Geometry: final body of the model. Coordinates: model frame, mm. A direction names the side the tool comes from. Coordinates: 2 decimals unless noted, no trailing zeros. Loops run counter-clockwise (first coordinate to the right, second up) from the corner with the lowest first, then second, coordinate; pieces in that order, holes last. Notation, with made-up numbers: (3.25, -5.75) -> (11.25, -5.75) arc R18 ccw to (11.25, 9.25) -> close; hole circle Ø10 at (-40, 4.25). An arc over 180 degrees is marked (long way). One line per item, written item: value. Start each with the question number.
Item 1: Ray query, probe 1 along Y at (x, z) = (252, -203); probe 2 along Z at (x, y) = (253.1, 44.45); probe 3 along Z at (x, y) = (-142, 14). Return the intervals inside material, ascending. Write a range as from..to.
Item 2: Set-up query: faces 1 (the flat face through (-504.952, 77, -186)), 2 (the flat face through (-508, 75, -186)). Return all of +Z, -Z, +X, -X, +Y, -Y with unobstructed straight access to the full face (end or side cutting, diameter ignored); none if empty.
Item 3: Section query B-B on x = -169.5. Return loops of the section in (y, z).
Item 4: Contact query for flat-ended pins moving along their axis: pin 1 Ø4 at (x, z) = (-195, -72) entering from +Y; pin 2 Ø7.5 at (y, z) = (44.45, -203.2) entering from +X; pin 3 Ø2.5 at (x, y) = (-117.348, 114.3) entering from -Z. Output: stop coordinate, or through.
Item 5: Section query C-C on z = -78. Return loops of the section in (x, y), then the cut area to 3 significant figures.
Item 6: Section query A-A on y = 124.5. Return loops of the section in (x, z).
Item 7: Mould query, pull axis X, two halves, no side actions, for faces 3 (the flat face through (-132, 0, -195)), 4 (the flat face through (-132, 77, 123.952)), 5 (the flat face through (254, 75, -186)). Classes: +X half, -X half, draft (parallel to the pull), parting line (faces both ways), or undercut.
from build123d import *

# Parameters (mm, degrees)
SKETCH1_W                          = 762
SKETCH1_H                          = 635
EXTRUDE1_DEPTH                     = 152.4
SHELL1_T                           = -3.048
SKETCH2_R                          = 6.35
CONNECTOR_MOUNT_CUT_EXTRUDE1_DEPTH = 929.403877631
LPATTERN1_START                    = -508
LPATTERN1_OUTLINE_R                = 6.35
LPATTERN1_DEPTH                    = 3.048
LPATTERN5_START                    = 250.952
LPATTERN5_OUTLINE_R                = 6.35
LPATTERN5_DEPTH                    = 3.048
SKETCH3_R                          = 1.524
CLIP_MOUNT_CUT_EXTRUDE2_DEPTH      = 39.624
LPATTERN2_COUNT                    = 5
LPATTERN2_PITCH                    = 101.6
LPATTERN2_COUNT_DIR2               = 2
LPATTERN2_PITCH_DIR2               = 63.5


# Read off the part's stored shape, not the designer's step: LPattern1, LPattern5
with BuildPart() as part:
    # Sketch1 → Extrude1 (new body)
    with BuildSketch(Plane(origin=(0, 0, 0), x_dir=(1, 0, 0), z_dir=(0, 1, 0))):
        with Locations((-127, 190.5)):
            Rectangle(SKETCH1_W, SKETCH1_H)
    extrude(amount=EXTRUDE1_DEPTH)

    # Shell1
    shell1_openings = [part.faces().sort_by_distance(p)[0] for p in [
        (-127, 152.4, -190.5),
    ]]
    offset(amount=SHELL1_T, openings=shell1_openings, kind=Kind.INTERSECTION)

    # Sketch2 → Connector mount--Cut-Extrude1 (cut, through all)
    with BuildSketch(Plane.ZY.offset(508)):
        with Locations((-406.4, 107.95)):
            Circle(SKETCH2_R)
    extrude(amount=-CONNECTOR_MOUNT_CUT_EXTRUDE1_DEPTH, mode=Mode.SUBTRACT)

    # LPattern1 outline → LPattern1 (cut)
    with BuildSketch(Plane.YZ.offset(LPATTERN1_START)):
        with Locations((107.95, 0)):
            Circle(LPATTERN1_OUTLINE_R)
        with Locations((107.95, -203.2)):
            Circle(LPATTERN1_OUTLINE_R)
    extrude(amount=LPATTERN1_DEPTH, mode=Mode.SUBTRACT)

    # LPattern5 outline → LPattern5 (cut)
    with BuildSketch(Plane.YZ.offset(LPATTERN5_START)):
        with Locations((44.45, 0)):
            Circle(LPATTERN5_OUTLINE_R)
        with Locations((44.45, -203.2)):
            Circle(LPATTERN5_OUTLINE_R)
        with Locations((44.45, -406.4)):
            Circle(LPATTERN5_OUTLINE_R)
        with Locations((107.95, 0)):
            Circle(LPATTERN5_OUTLINE_R)
        with Locations((107.95, -203.2)):
            Circle(LPATTERN5_OUTLINE_R)
    extrude(amount=LPATTERN5_DEPTH, mode=Mode.SUBTRACT)

    # Sketch3 → Clip Mount --Cut-Extrude2 (cut)
    with BuildSketch(Plane(origin=(0, 0, -508), x_dir=(-1, 0, 0), z_dir=(0, 0, -1))):
        with Locations((-85.852, 114.3)):
            Circle(SKETCH3_R)
    clip_mount_cut_extrude2 = extrude(amount=-CLIP_MOUNT_CUT_EXTRUDE2_DEPTH, mode=Mode.SUBTRACT)

    # LPattern2: Clip Mount --Cut-Extrude2 5 × 2, 6 skipped
    with Locations(*[(-i * LPATTERN2_PITCH, -j * LPATTERN2_PITCH_DIR2, 0) for i in range(LPATTERN2_COUNT) for j in range(LPATTERN2_COUNT_DIR2) if (i, j) not in ((0, 0), (0, 1), (1, 0), (1, 1), (2, 1), (3, 0), (4, 0))]):
        add(clip_mount_cut_extrude2, mode=Mode.SUBTRACT)


solid = part.part
Reply:
1. probe 1: y = 0..38.1, 50.8..101.6, 114.3..152.4
1. probe 2: z = -508..-412.75, -400.05..-209.55, -196.85..-6.35, 6.35..127
1. probe 3: z = -508..-504.95, 123.95..127
2. face 1: +Y
2. face 2: +Z, -Z, -X, +Y, -Y
3. outline: (0, -508) -> (152.4, -508) -> (152.4, -504.95) -> (3.05, -504.95) -> (3.05, 123.95) -> (152.4, 123.95) -> (152.4, 127) -> (0, 127) -> close
4. pin 1: stops at y = 3.05
4. pin 2: stops at x = -504.95
4. pin 3: stops at z = 123.95
5. outline: (-508, 0) -> (254, 0) -> (254, 152.4) -> (250.95, 152.4) -> (250.95, 3.05) -> (-504.95, 3.05) -> (-504.95, 152.4) -> (-508, 152.4) -> close
5. area: 3,230 mm²
6. outline: (-508, -508) -> (254, -508) -> (254, 127) -> (-508, 127) -> close; hole (-504.95, -504.95) -> (250.95, -504.95) -> (250.95, 123.95) -> (-504.95, 123.95) -> close
7. face 3: draft
7. face 4: undercut
7. face 5: +X half
